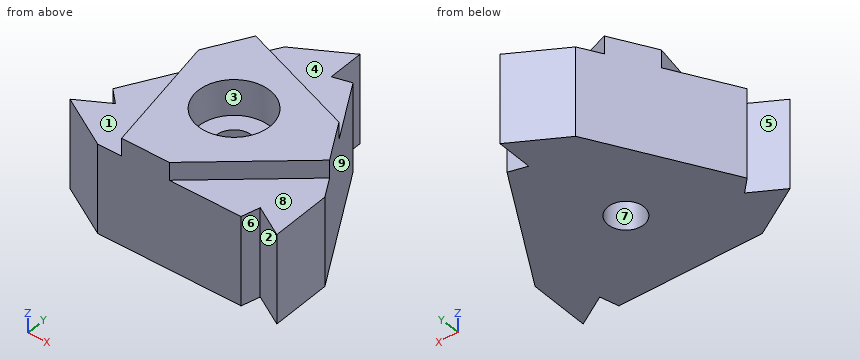
from build123d import *

# Parameters (mm, degrees)
EXTRUDE_1_DEPTH           = 9
CUT_EXTRUDE_5_DEPTH       = 1.5
HOLE_WIZARD_1_D           = 3
HOLE_WIZARD_1_CBORE_D     = 6
HOLE_WIZARD_1_CBORE_DEPTH = 3


with BuildPart() as part:
    # 草图1 → 凸台-拉伸1 (new body)
    with BuildSketch(Plane.XY):
        Polygon((-37.234772054, 15.490381057), (-43.234772054, 5.098076211), (-42.136695843, 4), (-44.734772054, 2.5), (-40.404645035, 0), (-28.404645035, 0), (-28.002721246, 1.5), (-25.404645035, 0), (-25.404645035, 5), (-31.404645035, 15.392304845), (-32.904645035, 14.990381057), (-32.904645035, 17.990381057), align=None)
    extrude(amount=EXTRUDE_1_DEPTH)

    # 草图2 → 切除-拉伸5 (cut)
    with BuildSketch(Plane.XY.offset(9)):
        Polygon((-38.404645035, 0), (-40.234772054, 10.294228634), (-43.234772054, 5.098076211), (-42.136695843, 4), (-44.734772054, 2.5), (-40.404645035, 0), align=None)
        Polygon((-38.234772054, 13.758330249), (-28.404645035, 10.196152423), (-31.404645035, 15.392304845), (-32.904645035, 14.990381057), (-32.904645035, 17.990381057), (-37.234772054, 15.490381057), align=None)
        Polygon((-26.404645035, 6.732050808), (-34.404645035, 0), (-28.404645035, 0), (-28.002721246, 1.5), (-25.404645035, 0), (-25.404645035, 5), align=None)
    extrude(amount=-CUT_EXTRUDE_5_DEPTH, mode=Mode.SUBTRACT)

    # 孔1 (through all)
    with Locations(Plane.XY.offset(9)):
        with Locations((-34.624141854, 7.012125204)):
            CounterBoreHole(HOLE_WIZARD_1_D / 2, HOLE_WIZARD_1_CBORE_D / 2, HOLE_WIZARD_1_CBORE_DEPTH)


solid = part.part
Geometry: final body of the model. Coordinates: model frame, mm. Face numbers are marked on the shaded views. A direction names the side the tool comes from. Give positions to 0.01 mm unless a question says otherwise; leave off trailing zeros. Loops run counter-clockwise (first coordinate to the right, second up) from the corner with the lowest first, then second, coordinate; pieces in that order, holes last. Notation, with made-up numbers: M 45,56.5 L 97,56.5 A7 ccw 97,62.5 Z; hole C 18.5,-20 d9. An arc over 180 degrees is marked long. Put each result on its own line as item: value. Start each with the question number.
1) Cut plane A-A (y = 1). Output: boundary loops of the cut face in (x, z).
2) Ray query, line 1 along Z through (x, y) = (-33.25, 8); line 2 along Z through (x, y) = (-41.75, 3.5); line 3 along X through (y, z) = (7, 5.75). Return the intervals inside material, ascending.
3) Access query for the marked faces 1, 2, 3, 4 and 5. Directions: +Z, -Z, +X, -X, +Y, -Y. A direction counts if a zero-diameter tool reaches every point of the face in a straight line with its end or side. Return the directions, or none.
4) Cut plane C-C (z = 6.5). Output: boundary loops of the cut face in (x, y), then the cut area to 3 significant figures.
5) Contact query for flat-ended pins moving along their axis: pin 1 (1.9 mm diameter, centred on x = -42, y = 4, fed in from +Z); pin 2 (1.8 mm diameter, centred on x = -34.5, y = 6, fed in from +Z); pin 3 (0.9 mm diameter, centred on y = 16.5, z = 4, fed in from +X). Output: stop coordinate, or through.
6) Cut plane D-D (x = -27.5). Output: boundary loops of the cut face in (y, z).
7) Pull-direction query (X, two-part tool) for the marked faces 6, 7, 8 and 9; classes: pulls with the +X half, pulls with the -X half, needs draft (parallel to the pull), parting line crosses it, or undercut.
8) Cut plane B-B (x = -35). Output: boundary loops of the cut face in (y, z), then the cut area to 3 significant figures.
Verdict:
1. outline: M -42.14,0 L -28.14,0 L -28.14,7.5 L -33.22,7.5 L -33.22,9 L -38.58,9 L -38.58,7.5 L -42.14,7.5 Z; M -27.14,0 L -25.4,0 L -25.4,7.5 L -27.14,7.5 Z
2. line 1: 0 to 6
2. line 2: 0 to 7.5
2. line 3: -42.14 to -36.12, -33.12 to -26.56
3. face 1: +Z, -X, -Y
3. face 2: +Z, -Z, -Y
3. face 3: +Z
3. face 4: +Z, +X, +Y
3. face 5: +Z, -Z, -X
4. outline: M -44.73,2.5 L -40.4,0 L -28.4,0 L -28,1.5 L -25.4,0 L -25.4,5 L -31.4,15.39 L -32.9,14.99 L -32.9,17.99 L -37.23,15.49 L -43.23,5.1 L -42.14,4 Z; hole C -34.62,7.01 d6
4. area: 186 mm2
5. pin 1: z = 7.5
5. pin 2: z = 6
5. pin 3: x = -32.9
6. outline: M 1.21,0 L 8.63,0 L 8.63,9 L 5.81,9 L 5.81,7.5 L 1.21,7.5 Z
7. face 6: undercut
7. face 7: undercut
7. face 8: needs draft
7. face 9: pulls with the +X half
8. outline: M 0,0 L 5.56,0 L 5.56,6 L 4.04,6 L 4.04,9 L 0,9 Z; M 8.46,0 L 16.78,0 L 16.78,7.5 L 12.59,7.5 L 12.59,9 L 9.99,9 L 9.99,6 L 8.46,6 Z
8. area: 109 mm2
